CAD build for the part. Positions are in the model's coordinates, mm. Face numbers are marked on the shaded views. Coordinates: 2 decimals unless noted, no trailing zeros. Order: outer loops, then holes, each group sorted by start corner. A loop starts at its lowest first (then second) coordinate and runs counter-clockwise, first axis right, second up. Notation, with made-up numbers: (35.25, 44) - (48.25, 44) arc R19 cw to (48.25, 66) - close; hole circle Ø7 at (8, -25.75). An arc over 180 degrees is marked (long way). Write each question's results on one line, items separated by ' | '. Start each with the question number.
Q1. Pull direction X, two halves, no side cores. Call the marked faces 1, 2 and 3: released by +X, released by -X, zero draft, split by the parting line, or undercut.
Q2. Pin check, flat tips, straight feed: P1, Ø1, axis at x = -4.5, z = 59, coming from the +Y side; P2, Ø10, axis at y = -13, z = 70.5, coming from the +X side; P3, Ø4, axis at x = 1, z = 55.5, coming from the +Y side. Stop position of each tip, or through.
Q3. Band-saw the part on A-A, the plane y = -34.5. Write the cut outline in (x, z) (3 decimals).
Q4. Band-saw the part on B-B, the plane z = 66. Write the cut outline in (x, y).
Q5. Band-saw the part on C-C, the plane x = -9.5. Write the cut outline in (y, z).
Q6. Band-saw the part on D-D, the plane y = -19. Write the cut outline in (x, z).
Q7. Wall check: probe 1 along Y at (x, z) = (-5.5, 96); probe 2 along Y at (x, z) = (-6.5, 49.5); probe 3 along X at (y, z) = (-3.5, 7). Give the ranges that are in metal, low to high.
```python
from build123d import *


with BuildPart() as f3:
    # F0 (on Top) → F3 section 0
    with BuildSketch(Plane.XY, mode=Mode.PRIVATE) as f3_s0:
        Polygon((-10.8, 11.85), (-39.6, 8.55), (-39.300002, -39.750002), (-6.6, -32.250002), (23.700001, -44.850003), (11.4, -20.250002), align=None)
    loft([f3_s0.sketch, Vertex(0, 0, 125)])


solid = f3.part
```
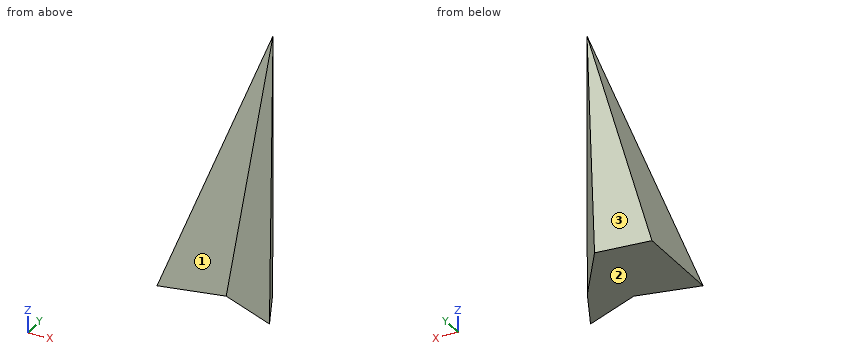
Results below:
1) face 1: undercut | face 2: zero draft | face 3: released by -X
2) P1: stops at y = 5.24 | P2: stops at x = 9.56 | P3: stops at y = -0.65
3) outline: (-39.333, 0) - (-16.41, 0) - (-34.109, 16.509) - close; (-1.189, 0) - (18.525, 0) - (18.231, 28.846) - close
4) outline: (-18.69, 4.04) - (-18.55, -18.76) - (-3.12, -15.22) - (11.19, -21.17) - (5.38, -9.56) - (-5.1, 5.59) - close
5) outline: (-32.92, 0) - (9.97, 0) - (10.42, 15.05) - (2.05, 95.01) - (-9.61, 94.78) - close
6) outline: (-39.43, 0) - (10.54, 0) - (10.7, 7.72) - (10.04, 72.05) - (-3.89, 51.36) - (-18.78, 65.25) - close
7) probe 1: y = -8.39 to 2.41 | probe 2: y = -20.06 to 7.12 | probe 3: x = -37.31 to -0.04
